Part model, mm, in its own coordinate system. Round coordinates to 2 decimals unless told otherwise and drop trailing zeros. Write each loop counter-clockwise with the first axis right and the second up, starting at its lowest first coordinate (ties: lowest second). Pieces come first, ordered by that corner, then holes.
1) Flat gauge pins, fed straight in: pin 1 (2 mm diameter, centred on x = 2, z = 24, fed in from -Y); pin 2 (2 mm diameter, centred on x = 1.5, z = 83.5, fed in from -Y); pin 3 (1.2 mm diameter, centred on x = 1.5, z = 25.5, fed in from +Y). Where does each tip first touch, or does it go through?
2) Drill centre lines: L1, parallel to Y at x = 1.9, z = 135; L2, parallel to Y at x = 3.65, z = 79; L3, parallel to Y at x = 2.6, z = 73. Where is each one in solid material? Low to high.
3) Saw through at A-A on x = 0.9. Write the cut outline in (y, z).
4) Saw through at C-C on z = 139. Write the cut outline in (x, y), and give its area (3 significant figures).
5) Saw through at D-D on z = 93. Write the cut outline in (x, y), and give its area (3 significant figures).
6) Saw through at B-B on z = 43. Write the cut outline in (x, y).
```python
from build123d import *

# Parameters (mm, degrees)
F0_R     = 4.25
F0_R_2   = 3.25
F1_DEPTH = 4
F2_R     = 25
F3_R     = 1


with BuildPart() as f1:
    # F0 (on Right) → F1 (new body)
    with BuildSketch(Plane.YZ):
        with BuildLine():
            ThreePointArc((-12.5, 0), (0, -12.5), (12.5, 0))
            Line((12.5, 0), (12.5, 50.003379))
            ThreePointArc((12.5, 50.003379), (20, 87), (12.5, 123.996621))
            Line((12.5, 123.996621), (12.5, 150))
            ThreePointArc((12.5, 150), (0, 162.5), (-12.5, 150))
            Line((-12.5, 150), (-12.5, 123.996621))
            ThreePointArc((-12.5, 123.996621), (-20, 87), (-12.5, 50.003379))
            Line((-12.5, 50.003379), (-12.5, 0))
        make_face()
        Circle(F0_R, mode=Mode.SUBTRACT)
        with Locations((0, 43)):
            Circle(F0_R_2, mode=Mode.SUBTRACT)
        with BuildLine():
            ThreePointArc((-4.25, 96.75), (-8.5, 101), (-4.25, 105.25))
            Line((-4.25, 105.25), (4.25, 105.25))
            ThreePointArc((4.25, 105.25), (7.255204, 104.005204), (8.5, 101))
            Line((8.5, 101), (8.5, 73))
            ThreePointArc((8.5, 73), (7.255204, 69.994796), (4.25, 68.75))
            Line((4.25, 68.75), (-4.25, 68.75))
            ThreePointArc((-4.25, 68.75), (-8.5, 73), (-4.25, 77.25))
            Line((-4.25, 77.25), (0, 77.25))
            Line((0, 77.25), (0, 96.75))
            Line((0, 96.75), (-4.25, 96.75))
        make_face(mode=Mode.SUBTRACT)
        with Locations((0, 150)):
            Circle(F0_R, mode=Mode.SUBTRACT)
    extrude(amount=F1_DEPTH)

    # F2
    f2_edges = [f1.edges().sort_by_distance(p)[0] for p in [
        (2, 12.5, 123.996621),
        (2, -12.5, 123.996621),
        (2, -12.5, 50.003379),
        (2, 12.5, 50.003379),
    ]]
    fillet(f2_edges, radius=F2_R)

    # F3
    f3_edges = [f1.edges().sort_by_distance(p)[0] for p in [
        (2, 0, 96.75),
        (2, 0, 77.25),
    ]]
    fillet(f3_edges, radius=F3_R)


solid = f1.part
```
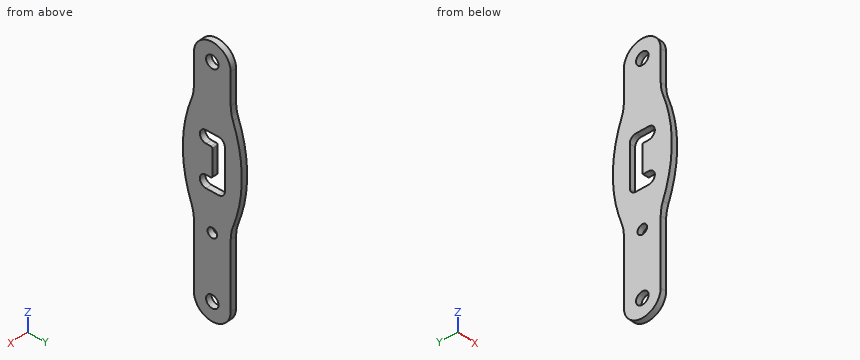
Completed:
1. pin 1: stops at y = -12.5
1. pin 2: stops at y = -19.97
1. pin 3: stops at y = 12.5
2. L1: y = -12.5 to 12.5
2. L2: y = -19.66 to 0, 8.5 to 19.66
2. L3: y = -18.96 to -8.5, 8.5 to 18.96
3. outline: (-14.06, 53.94) arc R25 cw to (-12.5, 45.24) - (-12.5, 0) arc R12.5 ccw to (12.5, 0) - (12.5, 45.24) arc R25 cw to (14.06, 53.94) arc R95 ccw to (14.06, 120.06) arc R25 cw to (12.5, 128.76) - (12.5, 150) arc R12.5 ccw to (-12.5, 150) - (-12.5, 128.76) arc R25 cw to (-14.06, 120.06) arc R95 ccw to start; hole circle Ø8.5 at (0, 0); hole (-4.25, 68.75) - (4.25, 68.75) arc R4.25 ccw to (8.5, 73) - (8.5, 101) arc R4.25 ccw to (4.25, 105.25) - (-4.25, 105.25) arc R4.25 ccw to (-4.25, 96.75) - (-1, 96.75) arc R1 cw to (0, 95.75) - (0, 78.25) arc R1 cw to (-1, 77.25) - (-4.25, 77.25) arc R4.25 ccw to start; hole circle Ø8.5 at (0, 150); hole circle Ø6.5 at (0, 43)
4. outline: (0, -12.5) - (4, -12.5) - (4, 12.5) - (0, 12.5) - close
4. area: 100 mm2
5. outline: (0, -19.81) - (4, -19.81) - (4, 0) - (0, 0) - close; (0, 8.5) - (4, 8.5) - (4, 19.81) - (0, 19.81) - close
5. area: 124 mm2
6. outline: (0, -12.5) - (4, -12.5) - (4, -3.25) - (0, -3.25) - close; (0, 3.25) - (4, 3.25) - (4, 12.5) - (0, 12.5) - close
